Read the model definition and answer for the solid it produces. Units are mm, in the model's axes. Face numbers are marked on the shaded views. A direction names the side the tool comes from. Give positions to 0.01 mm unless a question says otherwise; leave off trailing zeros. Write each loop counter-clockwise with the first axis right and the second up, starting at its lowest first coordinate (ties: lowest second). Pieces come first, ordered by that corner, then holes. Notation, with made-up numbers: (30.25, 52.25) - (53.25, 52.25) arc R31 cw to (53.25, 76.25) - close; hole circle Ø2 at (-29.5, -14). An arc over 180 degrees is marked (long way). Answer as CSV lines item,"result".
```python
from build123d import *

# Parameters (mm, degrees)
SALIENTE_EXTRUIR1_DEPTH = 10
CROQUIS2_R              = 1.9
CORTAR_EXTRUIR1_DEPTH   = 25
CROQUIS5_R              = 3.25
CORTAR_EXTRUIR3_DEPTH   = 4
CORTAR_EXTRUIR4_DEPTH   = 4.25
SALIENTE_EXTRUIR2_DEPTH = 25
CHAFL_N2_SIZE           = 6
SALIENTE_EXTRUIR3_DEPTH = 5
CROQUIS9_R              = 1.9
CORTAR_EXTRUIR5_DEPTH   = 62.56630572
CORTAR_EXTRUIR6_DEPTH   = 2.75
SALIENTE_EXTRUIR4_DEPTH = 0.2


with BuildPart() as part:
    # Croquis1 → Saliente-Extruir1 (new body)
    with BuildSketch(Plane.XY):
        with BuildLine():
            Line((51.5, 9.3), (-51.5, 9.3))
            ThreePointArc((-51.5, 9.3), (-55.742640687, 7.542640687), (-57.5, 3.3))
            Line((-57.5, 3.3), (-57.5, -3.3))
            ThreePointArc((-57.5, -3.3), (-55.742640687, -7.542640687), (-51.5, -9.3))
            Line((-51.5, -9.3), (-33.9, -9.3))
            Line((-33.9, -9.3), (-33.9, -1.5))
            Line((-33.9, -1.5), (-44.170111664, -1.5))
            ThreePointArc((-44.170111664, -1.5), (-52.5, 0), (-44.170111664, 1.5))
            Line((-44.170111664, 1.5), (-31.9, 1.5))
            Line((-31.9, 1.5), (-31.9, -9.3))
            Line((-31.9, -9.3), (31.9, -9.3))
            Line((31.9, -9.3), (31.9, 1.5))
            Line((31.9, 1.5), (44.170111664, 1.5))
            ThreePointArc((44.170111664, 1.5), (48.962063041, 4.231933355), (52.5, 0))
            ThreePointArc((52.5, 0), (48.962063041, -4.231933355), (44.170111664, -1.5))
            Line((44.170111664, -1.5), (33.9, -1.5))
            Line((33.9, -1.5), (33.9, -9.3))
            Line((33.9, -9.3), (51.5, -9.3))
            ThreePointArc((51.5, -9.3), (55.742640687, -7.542640687), (57.5, -3.3))
            Line((57.5, -3.3), (57.5, 3.3))
            ThreePointArc((57.5, 3.3), (55.742640687, 7.542640687), (51.5, 9.3))
        make_face()
    extrude(amount=SALIENTE_EXTRUIR1_DEPTH)

    # Croquis2 → Cortar-Extruir1 (cut, symmetric)
    with BuildSketch(Plane.XZ.offset(-1.5)):
        with Locations(Location((-39.035111664, 5, 0), (0, 0, 180))):
            Circle(CROQUIS2_R)
        with Locations(Location((39.035111664, 5, 0), (0, 0, 180))):
            Circle(CROQUIS2_R)
    extrude(amount=CORTAR_EXTRUIR1_DEPTH, both=True, mode=Mode.SUBTRACT)

    # Croquis5 → Cortar-Extruir3 (cut)
    with BuildSketch(Plane(origin=(0, 9.3, 0), x_dir=(1, 0, 0), z_dir=(0, 1, 0))):
        with Locations(Location((-39.035111664, -5, 0), (0, 0, 270))):
            Circle(CROQUIS5_R)
        with Locations(Location((39.035111664, -5, 0), (0, 0, 270))):
            Circle(CROQUIS5_R)
    extrude(amount=-CORTAR_EXTRUIR3_DEPTH, mode=Mode.SUBTRACT)

    # Croquis6 → Cortar-Extruir4 (cut)
    with BuildSketch(Plane(origin=(0, -9.3, 0), x_dir=(-1, 0, 0), z_dir=(0, -1, 0))):
        Polygon((42.499213279, -5), (40.767162472, -2), (37.303060857, -2), (35.571010049, -5), (37.303060857, -8), (40.767162472, -8), align=None)
        Polygon((-42.499213279, -5), (-40.767162472, -8), (-37.303060857, -8), (-35.571010049, -5), (-37.303060857, -2), (-40.767162472, -2), align=None)
    extrude(amount=-CORTAR_EXTRUIR4_DEPTH, mode=Mode.SUBTRACT)

    # Croquis7 → Saliente-Extruir2 (add, symmetric)
    with BuildSketch(Plane.ZY):
        Polygon((0, 9.3), (10, 15.3), (10, 12.3), (7, 9.3), align=None)
    extrude(amount=SALIENTE_EXTRUIR2_DEPTH, both=True)

    # Chaflán2
    # the kernel refuses this chamfer: 6 mm, written as the material it adds along each edge
    with BuildSketch(Plane(origin=(-25, 9.3, 22.430097928), x_dir=(-0.9996219169112968, -0.02749587661058678, 0), z_dir=(0, 0, -1))) as chafl_n2_piece_1_section:
        Polygon((CHAFL_N2_SIZE * 0.999621916911, CHAFL_N2_SIZE * 0.0274958766106), (-CHAFL_N2_SIZE * 0.0274958766106, CHAFL_N2_SIZE * 0.999621916911), (0, 0), align=None)
    chafl_n2_piece_1 = extrude(amount=37.860195856, mode=Mode.PRIVATE)
    chafl_n2_piece_1 = split(chafl_n2_piece_1, bisect_by=Plane(origin=(-27.180769231, 9.432692308, 7.132692308), z_dir=(0, 0.7071067811865436, -0.7071067811865516)), keep=Keep.TOP, mode=Mode.PRIVATE)
    chafl_n2_piece_1 = split(chafl_n2_piece_1, bisect_by=Plane(origin=(-27.180769231, 10.938461538, 10), z_dir=(0, 0, -1)), keep=Keep.TOP, mode=Mode.PRIVATE)
    chafl_n2_piece_1 = split(chafl_n2_piece_1, bisect_by=Plane(origin=(-27.180769231, 12.216176471, 4.860294118), z_dir=(0, -0.8574929257125441, 0.5144957554275267)), keep=Keep.TOP, mode=Mode.PRIVATE)
    add(chafl_n2_piece_1)
    with BuildSketch(Plane(origin=(25, 9.3, 22.430097928), x_dir=(0.9996219169112969, -0.02749587661058621, 0), z_dir=(0, 0, -1))) as chafl_n2_piece_2_section:
        Polygon((CHAFL_N2_SIZE * 0.999621916911, -CHAFL_N2_SIZE * 0.0274958766106), (-CHAFL_N2_SIZE * 0.0274958766106, -CHAFL_N2_SIZE * 0.999621916911), (0, 0), align=None)
    chafl_n2_piece_2 = extrude(amount=37.860195856, mode=Mode.PRIVATE)
    chafl_n2_piece_2 = split(chafl_n2_piece_2, bisect_by=Plane(origin=(27.180769231, 9.432692308, 7.132692308), z_dir=(0, 0.7071067811865436, -0.7071067811865516)), keep=Keep.TOP, mode=Mode.PRIVATE)
    chafl_n2_piece_2 = split(chafl_n2_piece_2, bisect_by=Plane(origin=(27.180769231, 10.938461538, 10), z_dir=(0, 0, -1)), keep=Keep.TOP, mode=Mode.PRIVATE)
    chafl_n2_piece_2 = split(chafl_n2_piece_2, bisect_by=Plane(origin=(27.180769231, 12.216176471, 4.860294118), z_dir=(0, -0.8574929257125441, 0.5144957554275267)), keep=Keep.TOP, mode=Mode.PRIVATE)
    add(chafl_n2_piece_2)

    # Croquis8 → Saliente-Extruir3 (add)
    with BuildSketch(Plane.XZ.offset(9.3)):
        with BuildLine():
            Line((-31.9, 0), (-35.941451884, -7))
            ThreePointArc((-35.941451884, -7), (-35.941451884, -9), (-34.209401077, -10))
            Line((-34.209401077, -10), (34.209401077, -10))
            ThreePointArc((34.209401077, -10), (35.941451884, -9), (35.941451884, -7))
            Line((35.941451884, -7), (31.9, 0))
            Line((31.9, 0), (-31.9, 0))
        make_face()
    extrude(amount=-SALIENTE_EXTRUIR3_DEPTH)

    # Croquis9 → Cortar-Extruir5 (cut, through all)
    with BuildSketch(Plane(origin=(0, -4.3, 0), x_dir=(1, 0, 0), z_dir=(0, 1, 0))):
        with Locations(Location((0, 4.5, 0), (0, 0, 180))):
            Circle(CROQUIS9_R)
        with Locations(Location((-29.498076211, 4.5, 0), (0, 0, 180))):
            Circle(CROQUIS9_R)
        with Locations(Location((-14.748076211, 4.5, 0), (0, 0, 180))):
            Circle(CROQUIS9_R)
        with Locations(Location((14.748076211, 4.5, 0), (0, 0, 180))):
            Circle(CROQUIS9_R)
        with Locations(Location((29.498076211, 4.5, 0), (0, 0, 180))):
            Circle(CROQUIS9_R)
    extrude(amount=-CORTAR_EXTRUIR5_DEPTH, mode=Mode.SUBTRACT)

    # Croquis10 → Cortar-Extruir6 (cut)
    with BuildSketch(Plane.XZ.offset(9.3)):
        Polygon((3.406366588, -4.5), (1.703183294, -1.55), (-1.703183294, -1.55), (-3.406366588, -4.5), (-1.703183294, -7.45), (1.703183294, -7.45), align=None)
        Polygon((-11.341709623, -4.5), (-13.044892917, -1.55), (-16.451259505, -1.55), (-18.1544428, -4.5), (-16.451259505, -7.45), (-13.044892917, -7.45), align=None)
        Polygon((-26.091709623, -4.5), (-27.794892917, -1.55), (-31.201259505, -1.55), (-32.9044428, -4.5), (-31.201259505, -7.45), (-27.794892917, -7.45), align=None)
        Polygon((18.1544428, -4.5), (16.451259505, -1.55), (13.044892917, -1.55), (11.341709623, -4.5), (13.044892917, -7.45), (16.451259505, -7.45), align=None)
        Polygon((32.9044428, -4.5), (31.201259505, -1.55), (27.794892917, -1.55), (26.091709623, -4.5), (27.794892917, -7.45), (31.201259505, -7.45), align=None)
    extrude(amount=-CORTAR_EXTRUIR6_DEPTH, mode=Mode.SUBTRACT)

    # Croquis11 → Saliente-Extruir4 (add)
    with BuildSketch(Plane(origin=(0, -4.3, 0), x_dir=(1, 0, 0), z_dir=(0, 1, 0))):
        Polygon((-31.9, 0), (-32.766025404, 1.5), (32.766025404, 1.5), (31.9, 0), align=None)
    extrude(amount=SALIENTE_EXTRUIR4_DEPTH)


solid = part.part
```
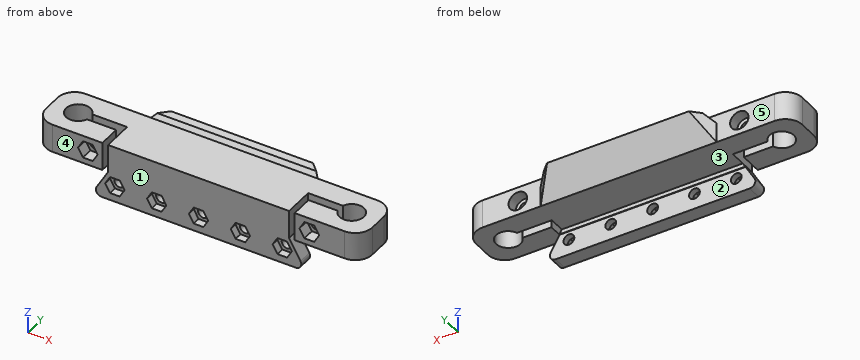
(1) A cutting plane is placed at A-A (x = -48.2). Write down the section's boundary in (y, z).
Worked out:
outline,"(-9.3, 0) - (-4.3, 0) - (-4.3, 10) - (-9.3, 10) - close; (4.3, 0) - (9.3, 0) - (9.3, 10) - (4.3, 10) - close"
(2) Each of these flat-tipped pins is pushed along its axis until it touches: P1, Ø1.5, axis at x = -31.5, z = -4.5, coming from the -Y side; P2, Ø5, axis at x = 39.5, z = 4, coming from the +Y side; P3, Ø3, axis at y = 9, z = 3, coming from the -X side. Where does it stop, or does it pass through?
Worked out:
P1,"stops at y = -6.55"
P2,"stops at y = 9.3"
P3,"stops at x = -55.78"
(3) A cutting plane is placed at B-B (y = 6.5). Write down the section's boundary in (x, z).
Worked out:
outline,"(-56.58, 0) - (56.58, 0) - (56.58, 10) - (-56.58, 10) - close; hole circle Ø6.5 at (-39.04, 5); hole circle Ø6.5 at (39.04, 5)"
(4) Find the intervals of material crossed by L1, parallel to X at y = 7.1, z = 5; L2, parallel to Y at x = 40.5, z = 8.75; L3, parallel to X at y = 6.5, z = 7.75, in increasing order.
Worked out:
L1,"x = -56.14 to -42.29, -35.79 to 35.79, 42.29 to 56.14"
L2,"y = -9.3 to -1.5, 1.5 to 9.3"
L3,"x = -56.58 to -40.77, -37.3 to 37.3, 40.77 to 56.58"
(5) The mould has two halves that part along Y. Classify the marked faces 3, 4 and 5: +Y half, -Y half, draft (parallel to the pull), parting line (faces both ways), or undercut.
Worked out:
face 3,"draft"
face 4,"-Y half"
face 5,"undercut"
(6) For the marked faces 1 and 2, determine the directions among +Z, -Z, +X, -X, +Y, -Y from which every point of the face is accessible in a straight line to the end or side of a thin tool.
Worked out:
face 1,"+Z, -Z, +X, -X, -Y"
face 2,"-Z, +X, -X, +Y"
(7) A cutting plane is placed at C-C (x = 0). Write down the section's boundary in (y, z), and give its area (3 significant figures).
Worked out:
outline,"(-9.3, -10) - (-4.3, -10) - (-4.3, -6.4) - (-6.55, -6.4) - (-6.55, -7.45) - (-9.3, -7.45) - close; (-9.3, -1.55) - (-6.55, -1.55) - (-6.55, -2.6) - (-4.3, -2.6) - (-4.3, -1.5) - (-4.1, -1.5) - (-4.1, 0) - (9.3, 0) - (15.3, 10) - (12.3, 10) - (9.3, 7) - (9.3, 10) - (-9.3, 10) - close"
area,"237 mm^2"
